Read the model definition and answer for the solid it produces. Units are mm, in the model's axes. Coordinates: 2 decimals unless noted, no trailing zeros. Write each loop counter-clockwise with the first axis right and the second up, starting at its lowest first coordinate (ties: lowest second). Pieces come first, ordered by that corner, then holes.
1) Find the intervals of material crossed by line 1 (X direction, y = 6, z = -24); line 2 (X direction, y = 6.25, z = -10.5); line 3 (X direction, y = 0.5, z = -148.5), in increasing order.
2) Each of these flat-tipped pins is pushed along its axis until it touches: pin 1 Ø3 at (y, z) = (1.5, -105) entering from +X; pin 2 Ø3 at (x, y) = (155, 1.5) entering from -Z; pin 3 Ø8 at (x, z) = (155, -27) entering from -Y. Where does it stop, or does it pass through?
3) The part is cut by section C-C (x = 91). Determine the outline of the cut face in (y, z), then the cut area to 3 significant figures.
4) The part is cut by section B-B (z = -182). Determine the outline of the cut face in (x, y).
5) The part is cut by section D-D (z = -23.5). Determine the outline of the cut face in (x, y).
6) The part is cut by section A-A (y = 1.75). Determine the outline of the cut face in (x, z), then the cut area to 3 significant figures.
from build123d import *

# Parameters (mm, degrees)
BOSS_EXTRUDE1_DEPTH = 6.35
FILLET1_R           = 12.7


with BuildPart() as part:
    # Sketch1 → Boss-Extrude1 (new body)
    with BuildSketch(Plane(origin=(0, 0, 0), x_dir=(1, 0, 0), z_dir=(0, 1, 0))):
        Polygon((74.847393185, 251.565850448), (-77.552606815, -12.398692626), (227.247393185, -12.398692626), align=None)
        with BuildLine():
            Line((68.624393185, 114.721772347), (72.434393185, 127.839947397))
            Line((72.434393185, 127.839947397), (72.434393185, 204.039947397))
            Line((72.434393185, 204.039947397), (77.260393185, 204.039947397))
            Line((77.260393185, 204.039947397), (77.260393185, 127.839947397))
            Line((77.260393185, 127.839947397), (81.070393185, 114.721772347))
            ThreePointArc((81.070393185, 114.721772347), (104.985753525, 101.313807865), (114.471393185, 75.589488399))
            ThreePointArc((114.471393185, 75.589488399), (113.810138601, 68.380754416), (111.848445192, 61.412622513))
            Line((111.848445192, 61.412622513), (121.304118037, 51.553978199))
            Line((121.304118037, 51.553978199), (187.295253805, 13.453978199))
            Line((187.295253805, 13.453978199), (184.882253805, 9.2745396))
            Line((184.882253805, 9.2745396), (118.891118037, 47.3745396))
            Line((118.891118037, 47.3745396), (105.625445192, 50.634070337))
            ThreePointArc((105.625445192, 50.634070337), (74.847393185, 35.965488399), (44.069341177, 50.634070337))
            Line((44.069341177, 50.634070337), (30.803668332, 47.3745396))
            Line((30.803668332, 47.3745396), (-35.187467436, 9.2745396))
            Line((-35.187467436, 9.2745396), (-37.600467436, 13.453978199))
            Line((-37.600467436, 13.453978199), (28.390668332, 51.553978199))
            Line((28.390668332, 51.553978199), (37.846341177, 61.412622512))
            ThreePointArc((37.846341177, 61.412622512), (40.532002585, 95.401488399), (68.624393185, 114.721772347))
        make_face(mode=Mode.SUBTRACT)
    extrude(amount=BOSS_EXTRUDE1_DEPTH)

    # Fillet1
    fillet1_edges = [part.edges().sort_by_distance(p)[0] for p in [
        (-77.552606815, 3.175, 12.398692626),
        (74.847393185, 3.175, -251.565850448),
        (227.247393185, 3.175, 12.398692626),
    ]]
    fillet(fillet1_edges, radius=FILLET1_R)


solid = part.part
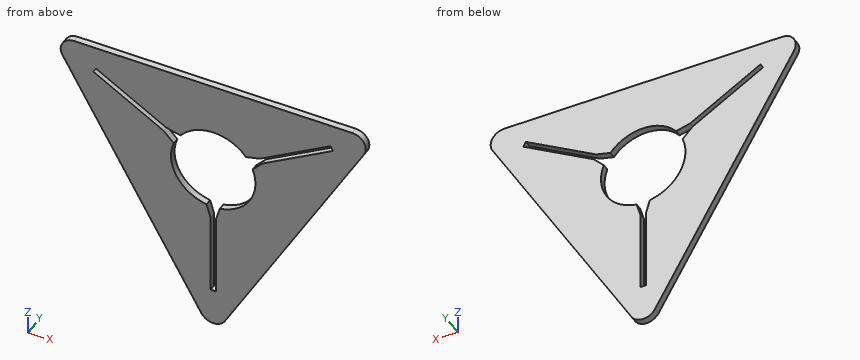
Reported:
1. line 1: x = -56.54 to -19.33, -9.68 to 159.38, 169.03 to 206.23
1. line 2: x = -64.33 to -35.89, -33.06 to 182.76, 185.59 to 214.03
1. line 3: x = 15.34 to 72.43, 77.26 to 134.35
2. pin 1: stops at x = 160.33
2. pin 2: stops at z = -115.34
2. pin 3: stops at y = 0
3. outline: (0, -223.59) - (6.35, -223.59) - (6.35, -111.77) - (0, -111.77) - close; (0, -39.41) - (6.35, -39.41) - (6.35, 12.4) - (0, 12.4) - close
3. area: 1,040 mm2
4. outline: (34.68, 0) - (72.43, 0) - (72.43, 6.35) - (34.68, 6.35) - close; (77.26, 0) - (115.01, 0) - (115.01, 6.35) - (77.26, 6.35) - close
5. outline: (-56.83, 0) - (-20.2, 0) - (-20.2, 6.35) - (-56.83, 6.35) - close; (-10.55, 0) - (160.24, 0) - (160.24, 6.35) - (-10.55, 6.35) - close; (169.9, 0) - (206.52, 0) - (206.52, 6.35) - (169.9, 6.35) - close
6. outline: (-66.55, -6.65) - (63.85, -232.52) arc R12.7 ccw to (85.85, -232.52) - (216.25, -6.65) arc R12.7 ccw to (205.25, 12.4) - (-55.56, 12.4) arc R12.7 ccw to start; hole (-37.6, -13.45) - (28.39, -51.55) - (37.85, -61.41) arc R39.62 ccw to (68.62, -114.72) - (72.43, -127.84) - (72.43, -204.04) - (77.26, -204.04) - (77.26, -127.84) - (81.07, -114.72) arc R39.62 ccw to (111.85, -61.41) - (121.3, -51.55) - (187.3, -13.45) - (184.88, -9.27) - (118.89, -47.37) - (105.63, -50.63) arc R39.62 ccw to (44.07, -50.63) - (30.8, -47.37) - (-35.19, -9.27) - close
6. area: 33,500 mm2
